from build123d import *

# Parameters (mm, degrees)
RESSALTO_EXTRUS_O1_DEPTH = 1.4
ESBO_O2_R                = 3.45
RESSALTO_EXTRUS_O2_DEPTH = 2.4
FURO4_D                  = 1.2
PADR_O_LINEAR1_COUNT     = 6
PADR_O_LINEAR1_PITCH     = 2
FURO1_D                  = 4.95
FURO1_DEPTH              = 2
FURO2_D                  = 4.6
FURO2_DEPTH              = 1
FURO3_D                  = 2.1
RESSALTO_EXTRUS_O3_DEPTH = 2
PADR_OCIRCULAR1_COUNT    = 60
CUT_EXTRUDE1_DEPTH       = 10
BOSS_EXTRUDE1_DEPTH      = 3.8
SKETCH4_W                = 22.5
SKETCH4_H                = 22.5
BOSS_EXTRUDE2_DEPTH      = 3.8
SKETCH5_R                = 6.1
SKETCH5_R_2              = 2.8
CUT_EXTRUDE2_DEPTH       = 10
SKETCH6_W                = 22.5
SKETCH6_H                = 8.135993376
BOSS_EXTRUDE3_DEPTH      = 8


with BuildPart() as part:
    # Esboço1 → Ressalto-extrusão1 (new body)
    with BuildSketch(Plane(origin=(0, 0, 0), x_dir=(1, 0, 0), z_dir=(0, 1, 0))):
        with BuildLine():
            Line((-14.159121967, 1.99702088), (-2.209072203, 2.65))
            ThreePointArc((-2.209072203, 2.65), (3.45, 0), (-2.209072203, -2.65))
            Line((-2.209072203, -2.65), (-14.159121967, -1.99702088))
            ThreePointArc((-14.159121967, -1.99702088), (-16.05, 0), (-14.159121967, 1.99702088))
        make_face()
    extrude(amount=-RESSALTO_EXTRUS_O1_DEPTH)

    # Esboço2 → Ressalto-extrusão2 (add)
    with BuildSketch(Plane.XZ.offset(1.4)):
        Circle(ESBO_O2_R)
    extrude(amount=RESSALTO_EXTRUS_O2_DEPTH)

    # Furo4 (through all)
    with Locations(Plane(origin=(0, 0, 0), x_dir=(1, 0, 0), z_dir=(0, 1, 0))):
        with Locations((-14.45, 0)):
            furo4 = Hole(FURO4_D / 2)

    # Padrão linear1: Furo4 ×6
    with Locations(*[(i * PADR_O_LINEAR1_PITCH, 0, 0) for i in range(1, PADR_O_LINEAR1_COUNT)]):
        add(furo4, mode=Mode.SUBTRACT)

    # Furo1
    with Locations(Plane(origin=(0, -3.8, 0), x_dir=(-1, 0, 0), z_dir=(0, -1, 0))):
        with Locations((0, 0)):
            Hole(FURO1_D / 2, depth=FURO1_DEPTH)

    # Furo2
    with Locations(Plane(origin=(0, 0, 0), x_dir=(1, 0, 0), z_dir=(0, 1, 0))):
        with Locations((0, 0)):
            Hole(FURO2_D / 2, depth=FURO2_DEPTH)

    # Furo3 (through all)
    with Locations(Plane(origin=(0, 0, 0), x_dir=(1, 0, 0), z_dir=(0, 1, 0))):
        with Locations((0, 0)):
            Hole(FURO3_D / 2)

    # Esboço11 → Ressalto-extrusão3 (add)
    with BuildSketch(Plane.XZ.offset(3.8)):
        with BuildLine():
            Line((-0.098056786, 2.473056786), (0, 2.375))
            Line((0, 2.375), (0.098056786, 2.473056786))
            ThreePointArc((0.098056786, 2.473056786), (0, 2.475), (-0.098056786, 2.473056786))
        make_face()
    ressalto_extrus_o3 = extrude(amount=-RESSALTO_EXTRUS_O3_DEPTH)

    # PadrãoCircular1: Ressalto-extrusão3 ×60 about axis
    padr_ocircular1_axis = Axis((0, 0, 0), (0, 1, 0))
    for i in range(1, PADR_OCIRCULAR1_COUNT):
        add(ressalto_extrus_o3.rotate(padr_ocircular1_axis, i * 360 / PADR_OCIRCULAR1_COUNT))

    # Sketch1 → Cut-Extrude1 (cut)
    with BuildSketch(Plane.XZ.offset(3.8)):
        with BuildLine():
            Line((0, 3.45), (-16.05, 3.45))
            Line((-16.05, 3.45), (-16.05, -3.45))
            Line((-16.05, -3.45), (0, -3.45))
            ThreePointArc((0, -3.45), (-3.45, 0), (0, 3.45))
        make_face()
    extrude(amount=-CUT_EXTRUDE1_DEPTH, mode=Mode.SUBTRACT)

    # Sketch2 → Boss-Extrude1 (add)
    with BuildSketch(Plane(origin=(0, 0, 0), x_dir=(1, 0, 0), z_dir=(0, 1, 0))):
        with BuildLine():
            Line((0, 3.45), (-11.841431407, 14.240980385))
            Line((-11.841431407, 14.240980385), (-11.841431407, 26.898431862))
            Line((-11.841431407, 26.898431862), (-1.20031972, 40.147481011))
            Line((-1.20031972, 40.147481011), (-5.293722372, 43.435139945))
            Line((-5.293722372, 43.435139945), (-17.141431407, 28.683779004))
            Line((-17.141431407, 28.683779004), (-17.141431407, 10.953171381))
            Line((-17.141431407, 10.953171381), (-2.323790008, -2.55))
            ThreePointArc((-2.323790008, -2.55), (-3.217141588, 1.245993579), (0, 3.45))
        make_face()
    extrude(amount=-BOSS_EXTRUDE1_DEPTH)

    # Sketch4 → Boss-Extrude2 (add)
    with BuildSketch(Plane.XZ.offset(3.8)):
        with Locations((0, 4.45)):
            Rectangle(SKETCH4_W, SKETCH4_H)
    extrude(amount=-BOSS_EXTRUDE2_DEPTH)

    # Sketch5 → Cut-Extrude2 (cut)
    with BuildSketch(Plane.XZ.offset(3.8)):
        Circle(SKETCH5_R)
        with Locations((0, 6.1)):
            Circle(SKETCH5_R_2)
    extrude(amount=-CUT_EXTRUDE2_DEPTH, mode=Mode.SUBTRACT)

    # Sketch6 → Boss-Extrude3 (add)
    with BuildSketch(Plane.XZ.offset(3.8)):
        with Locations((0, 19.767996688)):
            Rectangle(SKETCH6_W, SKETCH6_H)
    extrude(amount=-BOSS_EXTRUDE3_DEPTH)


solid = part.part
Verification items for the finished model (mm, model axes). A direction names the side the tool comes from. Coordinates: 2 decimals unless noted, no trailing zeros. Write each loop counter-clockwise with the first axis right and the second up, starting at its lowest first coordinate (ties: lowest second). Pieces come first, ordered by that corner, then holes. Notation, with made-up numbers: M -1.75,78 L 11.25,78 A6 cw 11.25,88 Z; hole C -13,-6.5 d11. An arc over 180 degrees is marked long. Use a Markdown table: item, result.
Q1. Draft check along X on faces 4 (the face through (0.1, -1.9, 8.9)), 5 (the face through (-11.25, -2, 12)), 6 (the face through (-11.841, -2, -20)). Enter one of: +X half, -X half, draft (parallel to the pull), parting line (faces both ways), or undercut.
Reply:
| item | result |
|---|---|
| face 4 | undercut |
| face 5 | -X half |
| face 6 | +X half |
Q2. Sectioned sample at B-B, the plane x = 0. Record the boundary of the cut face in (y, z).
Reply:
| item | result |
|---|---|
| outline | M -3.8,-6.8 L 0,-6.8 L 0,-6.1 L -3.8,-6.1 Z; M -3.8,8.9 L 0,8.9 L 0,15.7 L 4.2,15.7 L 4.2,23.84 L -3.8,23.84 Z |
Q3. Set-up check for faces 1 (the face through (4, -2, -6.8)), 2 (the face through (-17.141, -2, -20)), 3 (the face through (-6, 0, -8)): record each of +Z, -Z, +X, -X, +Y, -Y from which the full face is reachable in a straight line by a thin tool's end or side.
Reply:
| item | result |
|---|---|
| face 1 | +X, +Y, -Y |
| face 2 | +Z, -Z, -X, +Y, -Y |
| face 3 | -Z, +X, -X, +Y |
Q4. Sectioned sample at A-A, the plane z = 6.1. Record the boundary of the cut face in (x, y), plus the area to 3 significant figures.
Reply:
| item | result |
|---|---|
| outline | M -11.25,-3.8 L -2.8,-3.8 L -2.8,0 L -11.25,0 Z; M 2.8,-3.8 L 11.25,-3.8 L 11.25,0 L 2.8,0 Z |
| area | 64.2 mm² |
Q5. Go/stop test with flat-tipped pins: P1, Ø4, axis at y = 0, z = -7, coming from the +X side; P2, Ø1.9, axis at y = -2, z = -19, coming from the +X side; P3, Ø8.5, axis at x = -9, z = -2.5, coming from the +Y side; P4, Ø4, axis at x = -11.5, y = -0.5, coming from the -Z side. Record where each tip stops, or that it passes through.
Reply:
| item | result |
|---|---|
| P1 | stops at x = 11.25 |
| P2 | stops at x = -11.84 |
| P3 | stops at y = 0 |
| P4 | stops at z = -38.2 |
Q6. Sectioned sample at C-C, the plane y = -2.5. Record the boundary of the cut face in (x, z).
Reply:
| item | result |
|---|---|
| outline | M -17.14,-28.68 L -5.29,-43.44 L -1.2,-40.15 L -11.84,-26.9 L -11.84,-14.24 L -3.68,-6.8 L 11.25,-6.8 L 11.25,23.84 L -11.25,23.84 L -11.25,-5.58 L -17.14,-10.95 Z; hole M -2.73,5.46 A6.1 ccw long 2.73,5.46 A2.8 ccw long Z |
Q7. Sectioned sample at D-D, the plane x = -8.75. Record the boundary of the cut face in (y, z), plus the area to 3 significant figures.
Reply:
| item | result |
|---|---|
| outline | M -3.8,-39.13 L 0,-39.13 L 0,-30.75 L -3.8,-30.75 Z; M -3.8,-11.42 L 0,-11.42 L 0,15.7 L 4.2,15.7 L 4.2,23.84 L -3.8,23.84 Z |
| area | 200 mm² |
Q8. Thickness scan on line 1 (Z direction, x = 0, y = -2.7); line 2 (X direction, y = -2.3, z = 6.1); line 3 (X direction, y = -0.9, z = 0). Record the ranges inside material, lowest first.
Reply:
| item | result |
|---|---|
| line 1 | z = -6.8 to -6.1, 8.9 to 23.84 |
| line 2 | x = -11.25 to -2.8, 2.8 to 11.25 |
| line 3 | x = -11.25 to -6.1, 6.1 to 11.25 |
